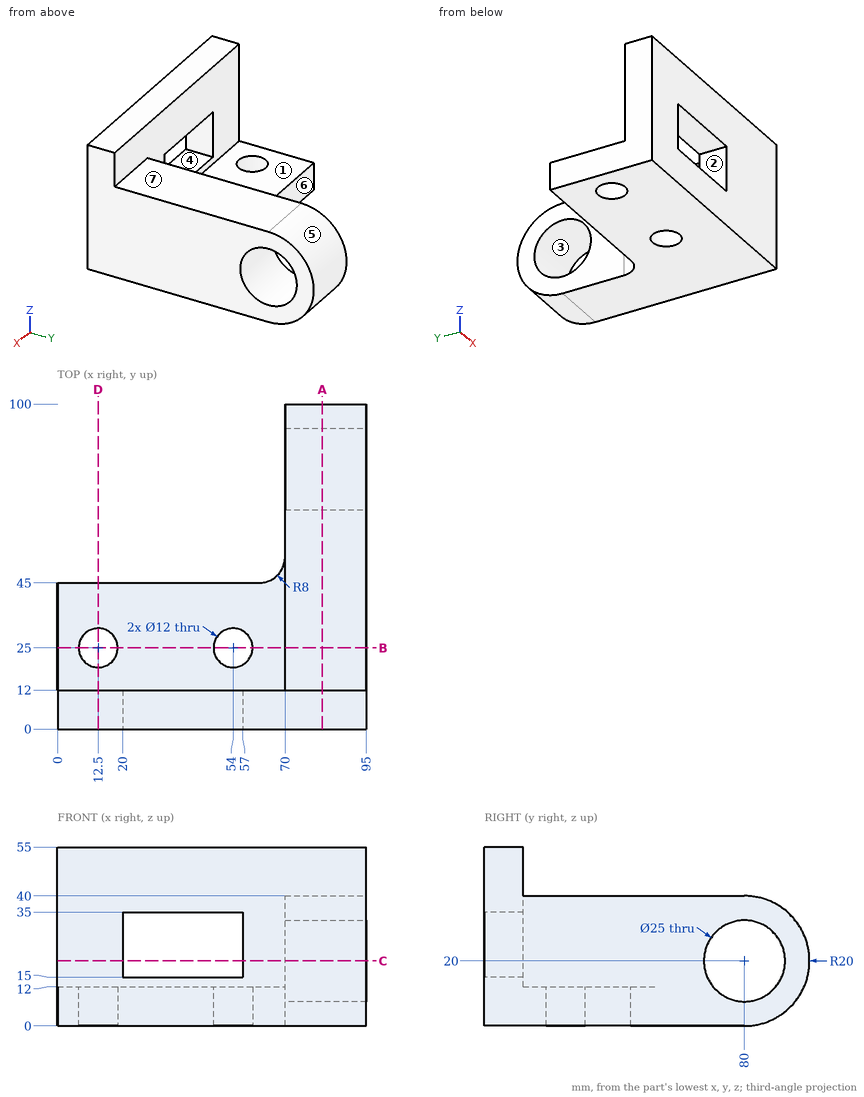
Study the drawing (mm; zero at the part's minimum x, y, z) and answer. A direction names the side the tool comes from. Give positions to 0.01 mm unless a question says otherwise; leave off trailing zeros. Write each loop counter-clockwise with the first axis right and the second up, starting at its lowest first coordinate (ties: lowest second). Pieces come first, ordered by that corner, then holes. Notation, with made-up numbers: M 78,16 L 126,16 A14 cw 126,36 Z; hole C 53.5,30.25 d7. An arc over 180 degrees is marked long. Put each result on its own line as item: value. Start each with the question number.
1. The part is cut by section B-B, the plane y = 25. Give the vertices of the cut face in (x, z).
2. Which of the six approach directions +Z, -Z, +X, -X, +Y, -Y give full straight-line access (tool end or side, diameter ignored) to the marked faces 1, 2 and 3?
3. The part is cut by section A-A, the plane x = 81.5. Give the vertices of the cut face in (y, z), and give its area (3 significant figures).
4. For a pull along Z with two mould halves and no side action, classify the marked faces 4, 5, 6 and 7 as released by +Z, released by -Z, zero draft, split by the parting line, or undercut.
5. The part is cut by section C-C, the plane z = 20. Give the vertices of the cut face in (x, y).
6. Each of these flat-tipped pins is pushed along its axis until it touches: pin 1 Ø2 at (x, z) = (85, 39.5) entering from +Y; pin 2 Ø9.5 at (x, y) = (54, 25) entering from +Z; pin 3 Ø7.5 at (x, y) = (77, 54.5) entering from +Z; pin 4 Ø3 at (x, y) = (43.5, 37) entering from +Z. Where does it stop, or does it pass through?
7. The part is cut by section D-D, the plane x = 12.5. Give the vertices of the cut face in (y, z), and give its area (3 significant figures).
8. Consider line 1 along Y through (x, z) = (12.5, 4.25); line 2 along X through (y, z) = (6, 27); line 3 along Y through (x, z) = (85.5, 20). Determine where each line is inside the solid, lowest interval first.
Final values:
1. outline: M 0,0 L 6.5,0 L 6.5,12 L 0,12 Z; M 18.5,0 L 48,0 L 48,12 L 18.5,12 Z; M 60,0 L 95,0 L 95,40 L 70,40 L 70,12 L 60,12 Z
2. face 1: +Z, -X, +Y
2. face 2: +Y, -Y
2. face 3: +X, -X
3. outline: M 0,0 L 80,0 A20 ccw 80,40 L 12,40 L 12,55 L 0,55 Z; hole C 80,20 d25
3. area: 3,520 mm²
4. face 4: undercut
4. face 5: split by the parting line
4. face 6: zero draft
4. face 7: released by +Z
5. outline: M 0,0 L 20,0 L 20,12 L 0,12 Z; M 57,0 L 95,0 L 95,67.5 L 70,67.5 L 70,12 L 57,12 Z; M 70,92.5 L 95,92.5 L 95,100 L 70,100 Z
6. pin 1: stops at y = 87.6
6. pin 2: passes through
6. pin 3: stops at z = 40
6. pin 4: stops at z = 12
7. outline: M 0,0 L 19,0 L 19,12 L 12,12 L 12,55 L 0,55 Z; M 31,0 L 45,0 L 45,12 L 31,12 Z
7. area: 912 mm²
8. line 1: y = 0 to 19, 31 to 45
8. line 2: x = 0 to 20, 57 to 95
8. line 3: y = 0 to 67.5, 92.5 to 100
